```python
from build123d import *

# Parameters (mm, degrees)
BOSS_EXTRUDE1_DEPTH = 12.7


with BuildPart() as part:
    # Sketch1 → Boss-Extrude1 (new body)
    with BuildSketch(Plane(origin=(0, 0, 0), x_dir=(1, 0, 0), z_dir=(0, 1, 0))):
        with BuildLine():
            Line((3.666174209, -6.35), (19.05, -6.35))
            Line((19.05, -6.35), (19.05, -3.175))
            Line((19.05, -3.175), (9.810775982, 8.064655891))
            ThreePointArc((9.810775982, 8.064655891), (0, 12.7), (-9.810775982, 8.064655891))
            Line((-9.810775982, 8.064655891), (-19.05, -3.175))
            Line((-19.05, -3.175), (-19.05, -6.35))
            Line((-19.05, -6.35), (-3.666174209, -6.35))
            Line((-3.666174209, -6.35), (-7.332348419, 0))
            Line((-7.332348419, 0), (-3.666174209, 6.35))
            Line((-3.666174209, 6.35), (3.666174209, 6.35))
            Line((3.666174209, 6.35), (7.332348419, 0))
            Line((7.332348419, 0), (3.666174209, -6.35))
        make_face()
    extrude(amount=BOSS_EXTRUDE1_DEPTH)


solid = part.part
```
Geometry check sheet. Reference: the model listing, model coordinates, mm. A direction names the side the tool comes from. Round coordinates to 2 decimals unless told otherwise and drop trailing zeros. Order: outer loops, then holes, each group sorted by start corner. A loop starts at its lowest first (then second) coordinate and runs counter-clockwise, first axis right, second up. Notation, with made-up numbers: M 6,58.5 L 31,58.5 A16 ccw 31,87.5 Z; hole C 21,-11 d5. An arc over 180 degrees is marked long. Answer as CSV lines item,"result".
1) Gauge pin test, flat ends, axial feed: pin 1 Ø1.5 at (y, z) = (4, -0.5) entering from -X; pin 2 Ø4 at (y, z) = (3, -1.5) entering from -X; pin 3 Ø5 at (y, z) = (5, -9) entering from -X. Record the tip position at first contact, or that the pin passes through.
Entries:
pin 1,"x = -16.65"
pin 2,"x = -16.85"
pin 3,"x = -11.1"
2) Tool access check on faces 1 (the face through (0, 6, -6.35)), 2 (the face through (5.474, 6.261, -3.219)), 3 (the face through (19.05, 6, 5)). Record the directions out of +Z, -Z, +X, -X, +Y, -Y that give a thin tool (end or side, any length) a straight path to the whole face; none if there is none.
Entries:
face 1,"+Z, +Y, -Y"
face 2,"+Y, -Y"
face 3,"+Z, -Z, +X, +Y, -Y"
3) Mould release check, pull along X, two halves, no side actions. Record for faces 4 (the face through (5.525, 6.261, 3.131)), 5 (the face through (14.495, 6.261, -2.366)), 6 (the face through (-5, 12.7, -5)), 7 (the face through (-5.474, 6.261, 3.219)): +X half, -X half, draft (parallel to the pull), parting line (faces both ways), or undercut.
Entries:
face 4,"undercut"
face 5,"+X half"
face 6,"draft"
face 7,"undercut"
4) Sectioned sample at A-A on z = 4.75. Record the cut outline in (x, y), and give its area (3 significant figures).
Entries:
outline,"M -19.05,0 L -4.59,0 L -4.59,12.7 L -19.05,12.7 Z; M 4.59,0 L 19.05,0 L 19.05,12.7 L 4.59,12.7 Z"
area,"367 mm2"
5) Thickness scan on probe 1 along Z at (x, y) = (-4.5, 4); probe 2 along X at (y, z) = (6.5, 0); probe 3 along X at (y, z) = (5, -5.25). Record the ranges inside material, lowest first. Write a range as [from, to].
Entries:
probe 1,"[-11.88, -4.91], [4.91, 6.35]"
probe 2,"[-16.44, -7.33], [7.33, 16.44]"
probe 3,"[-12.12, -4.3], [4.3, 12.12]"
6) Sectioned sample at D-D on z = -9. Record the cut outline in (x, y).
Entries:
outline,"M -8.96,0 L 8.96,0 L 8.96,12.7 L -8.96,12.7 Z"
7) Sectioned sample at B-B on y = 10.5. Record the cut outline in (x, z) (3 decimals).
Entries:
outline,"M -19.05,3.175 L -9.811,-8.065 A12.7 ccw 9.811,-8.065 L 19.05,3.175 L 19.05,6.35 L 3.666,6.35 L 7.332,0 L 3.666,-6.35 L -3.666,-6.35 L -7.332,0 L -3.666,6.35 L -19.05,6.35 Z"
8) Sectioned sample at C-C on z = -2.5. Record the cut outline in (x, y).
Entries:
outline,"M -14.39,0 L -5.89,0 L -5.89,12.7 L -14.39,12.7 Z; M 5.89,0 L 14.39,0 L 14.39,12.7 L 5.89,12.7 Z"
